from build123d import *

# Parameters (mm, degrees)
SKETCH1_W           = 254
SKETCH1_H           = 419.1
BOSS_EXTRUDE1_DEPTH = 368.3
CHAMFER1_SIZE       = 101.6
CHAMFER1_SIZE2      = 36.979375801
FILLET1_R           = 50.8
SKETCH2_R           = 6.35
BOSS_EXTRUDE2_DEPTH = 50.8
FILLET2_R           = 38.1
FILLET3_R           = 38.1


with BuildPart() as part:
    # Sketch1 → Boss-Extrude1 (new body)
    with BuildSketch(Plane(origin=(0, 0, 0), x_dir=(1, 0, 0), z_dir=(0, 1, 0))):
        Rectangle(SKETCH1_W, SKETCH1_H)
    extrude(amount=BOSS_EXTRUDE1_DEPTH)

    # Chamfer1
    chamfer1_edges = [part.edges().sort_by_distance(p)[0] for p in [
        (0, 368.3, 209.55),
    ]]
    chamfer1_side = [part.faces().sort_by_distance(p)[0] for p in [
        (0, 184.15, 209.55),
    ]]
    chamfer(chamfer1_edges, length=CHAMFER1_SIZE, length2=CHAMFER1_SIZE2, reference=chamfer1_side[0])

    # Fillet1
    fillet1_edges = [part.edges().sort_by_distance(p)[0] for p in [
        (0, 368.3, 172.570624199),
        (0, 266.7, 209.55),
    ]]
    fillet(fillet1_edges, radius=FILLET1_R)

    # Sketch2 → Boss-Extrude2 (add)
    with BuildSketch(Plane(origin=(0, 368.3, 0), x_dir=(1, 0, 0), z_dir=(0, 1, 0))):
        with Locations(Location((-50.8, 152.4, 0), (0, 0, 270))):
            Circle(SKETCH2_R)
        with Locations(Location((50.8, 152.4, 0), (0, 0, 270))):
            Circle(SKETCH2_R)
    extrude(amount=BOSS_EXTRUDE2_DEPTH)

    # Fillet2
    fillet2_edges = [part.edges().sort_by_distance(p)[0] for p in [
        (-127, 368.3, -36.274959371),
        (127, 128.87129469, 209.55),
        (-127, 128.87129469, 209.55),
        (-127, 304.995917971, 195.611425765),
        (-127, 359.11292385, 166.137764224),
        (-127, 266.563916805, 208.778233853),
        (127, 304.995917971, 195.611425765),
        (127, 368.3, -36.274959371),
        (127, 359.11292385, 166.137764224),
        (127, 266.563916805, 208.778233853),
    ]]
    fillet(fillet2_edges, radius=FILLET2_R)

    # Fillet3
    fillet3_edges = [part.edges().sort_by_distance(p)[0] for p in [
        (0, 368.3, -209.55),
        (-127, 165.1, -209.55),
        (127, 165.1, -209.55),
        (115.840768363, 357.140768363, -209.55),
        (-115.840768363, 357.140768363, -209.55),
    ]]
    fillet(fillet3_edges, radius=FILLET3_R)


solid = part.part
Could you check a few things on this model? Use its own coordinates, in mm. A direction names the side the tool comes from. Give positions to 0.01 mm unless a question says otherwise; leave off trailing zeros. Order: outer loops, then holes, each group sorted by start corner. A loop starts at its lowest first (then second) coordinate and runs counter-clockwise, first axis right, second up.
1. Suppose I cut it at C-C (x = 50.8). List the corners of the cut face in (y, z) for me.
2. I need wall thicknesses on L1, parallel to Y at x = 42.5, z = -22.5; L2, parallel to Y at x = 27, z = 175.5; L3, parallel to X at y = 68, z = 186.5. Which ranges of each line are inside material? Lowest first, please.
3. Suppose I cut it at D-D (z = -29). List the corners of the cut face in (x, y) for me.
4. Will these pins go through, and if not, where does the flat tip stop? P1, Ø6, axis at x = 13, y = 344, coming from the +Z side; P2, Ø1.5, axis at x = 92.5, y = 337.5, coming from the -Z side; P3, Ø1.5, axis at x = -63.5, z = -12, coming from the -Y side; P4, Ø6, axis at x = -60.5, z = 143.5, coming from the +Y side.
5. We'd pull the mould along X, two halves only. Please class faces 3 (the flat face through (-1.24, 305.41, 195.46)), 4 (the cylindrical face through (52.707, 393.344, -146.343)), 5 (the cylindrical face through (-116.14, 356.84, -19.38)): pulls with the +X half, pulls with the -X half, needs draft (parallel to the pull), parting line crosses it, or undercut.
6. Suppose I cut it at B-B (x = -27.5). List the corners of the cut face in (y, z) for me, plus the area to 3 significant figures.
7. For faces 1 (the cylindrical face through (-115.54, 167.41, -198.69)), 2 (the cylindrical face through (-48.893, 393.344, -146.343)), which set-ups out of +Z, -Z, +X, -X, +Y, -Y let a thin tool reach every point of the face, with its end or its side?
8. Suppose I cut it at A-A (z = -152.4). List the corners of the cut face in (x, y) for me.
Solved:
1. outline: (0, -209.55) - (330.2, -209.55) arc R38.1 ccw to (368.3, -171.45) - (368.3, -158.75) - (419.1, -158.75) - (419.1, -146.05) - (368.3, -146.05) - (368.3, 137) arc R50.8 ccw to (334.87, 184.74) - (275.12, 206.49) arc R50.8 ccw to (257.74, 209.55) - (0, 209.55) - close
2. L1: y = 0 to 368.3
2. L2: y = 0 to 350.64
2. L3: x = -123.9 to 123.9
3. outline: (-127, 0) - (127, 0) - (127, 330.2) arc R38.1 ccw to (88.9, 368.3) - (-88.9, 368.3) arc R38.1 ccw to (-127, 330.2) - close
4. P1: stops at z = 182.04
4. P2: stops at z = -208.83
4. P3: stops at y = 0
4. P4: stops at y = 368.18
5. face 3: needs draft
5. face 4: undercut
5. face 5: pulls with the -X half
6. outline: (0, -209.55) - (330.2, -209.55) arc R38.1 ccw to (368.3, -171.45) - (368.3, 137) arc R50.8 ccw to (334.87, 184.74) - (275.12, 206.49) arc R50.8 ccw to (257.74, 209.55) - (0, 209.55) - close
6. area: 152,000 mm2
7. face 1: -Z, -X, +Y, -Y
7. face 2: +Y
8. outline: (-127, 0) - (127, 0) - (127, 330.2) arc R38.1 ccw to (88.9, 368.3) - (57.15, 368.3) - (57.15, 419.1) - (44.45, 419.1) - (44.45, 368.3) - (-44.45, 368.3) - (-44.45, 419.1) - (-57.15, 419.1) - (-57.15, 368.3) - (-88.9, 368.3) arc R38.1 ccw to (-127, 330.2) - close
